```python
from build123d import *

# Parameters (mm, degrees)
F0_R     = 6
F1_DEPTH = 25
F3_DEPTH = 12.5


with BuildPart() as f1:
    # F0 (on Front) → F1 (new body)
    with BuildSketch(Plane.XZ):
        with BuildLine():
            ThreePointArc((-30.709658, -8), (-28.560439, -4.253905), (-27.814344, 0))
            ThreePointArc((-27.814344, 0), (-28.560439, 4.253905), (-30.709658, 8))
            ThreePointArc((-30.709658, 8), (-52.814344, 0), (-30.709658, -8))
        make_face()
        with Locations((-40.314344, 0)):
            Circle(F0_R, mode=Mode.SUBTRACT)
        with BuildLine():
            ThreePointArc((-30.709658, 8), (-28.560439, 4.253905), (-27.814344, 0))
            ThreePointArc((-27.814344, 0), (-28.560439, -4.253905), (-30.709658, -8))
            Line((-30.709658, -8), (38.685656, -8))
            ThreePointArc((38.685656, -8), (34.685656, 0), (38.685656, 8))
            Line((38.685656, 8), (-30.709658, 8))
        make_face()
        with BuildLine():
            ThreePointArc((54.685656, 0), (49.157792, 8.944272), (38.685656, 8))
            ThreePointArc((38.685656, 8), (34.685656, 0), (38.685656, -8))
            ThreePointArc((38.685656, -8), (49.157792, -8.944272), (54.685656, 0))
        make_face()
        with Locations((44.685656, 0)):
            Circle(F0_R, mode=Mode.SUBTRACT)
    extrude(amount=F1_DEPTH)

    # F2 (on Top) → F3 (intersect, symmetric)
    with BuildSketch(Plane.XY):
        Polygon((-51.041536, -9), (-52.814344, -9), (-52.814344, -17), (-50.341627, -17), (0.699909, -8), (54.685656, -8), (54.685656, 0), (25.572881, 0), (0, 0), align=None)
    extrude(amount=F3_DEPTH, both=True, mode=Mode.INTERSECT)


solid = f1.part
```
CAD build for the part. Positions are in the model's coordinates, mm. A direction names the side the tool comes from. Give positions to 0.01 mm unless a question says otherwise; leave off trailing zeros. Order: outer loops, then holes, each group sorted by start corner. A loop starts at its lowest first (then second) coordinate and runs counter-clockwise, first axis right, second up.
(1) Saw through at C-C, the plane y = -2.5. Give the cut face in (x, z), then the cut area to 3 significant figures.
(2) Flat gauge pins, fed straight in: pin 1 (8 mm diameter, centred on x = 12.5, z = -6.5, fed in from -Y); pin 2 (2 mm diameter, centred on x = -51.5, z = -2, fed in from +Y); pin 3 (2 mm diameter, centred on x = -19, y = -7, fed in from +Z). Where does each tip first touch, or does it go through?
(3) Drill centre lines: L1, parallel to Z at x = -40.5, y = -9.75; L2, parallel to Y at x = 4.5, z = -6.25; L3, parallel to Z at x = 9, y = -6.25. Where is each one in solid material? Low to high.
(4) Mould opens along X. For faces 6 (the flat face through (4, -5, -8)), 7 (the flat face through (-25.163, -4.437, 0.175)), 8 (the flat face through (27, 0, 0)) say: released by +X, released by -X, zero draft, split by the parting line, or undercut.
(5) Saw through at A-A, the plane y = -11. Give the cut face in (x, z).
(6) Saw through at B-B, the plane x = 6. Give the cut face in (y, z).
(7) Tool access for faces 1 (the flat face through (-51, -17, 0)), 2 (the cylindrical face through (-52.807, -11.126, 0.428)), 3 (the flat face through (27, -8, 0)), 4 (the flat face through (-52, -9, 0)), 5 (the flat face through (4, -5, 8)): list every direction of +Z, -Z, +X, -X, +Y, -Y with a clear straight run to the whole face (end or side of a thin tool).
Results found:
1. outline: (-14.18, -8) - (38.69, -8) arc R10 ccw (long way) to (38.69, 8) - (-14.18, 8) - close; hole circle Ø12 at (44.69, 0)
1. area: 1,000 mm2
2. pin 1: stops at y = -8
2. pin 2: stops at y = -8.9
2. pin 3: stops at z = 8
3. L1: z = -12.5 to -6, 6 to 12.5
3. L2: y = -8 to 0
3. L3: z = -8 to 8
4. face 6: undercut
4. face 7: released by -X
4. face 8: zero draft
5. outline: (-30.71, -8) - (-16.31, -8) - (-16.31, 8) - (-30.71, 8) arc R12.5 ccw (long way) to start; hole circle Ø12 at (-40.31, 0)
6. outline: (-8, -8) - (0, -8) - (0, 8) - (-8, 8) - close
7. face 1: +Z, -Z, +X, -X, -Y
7. face 2: +Y, -Y
7. face 3: +Z, -Z, +X, -Y
7. face 4: +Z, -Z, -X, +Y
7. face 5: +Z, +Y, -Y
